```python
from build123d import *

# Parameters (mm, degrees)
F0_R      = 10
F1_DEPTH  = 5
F2_W      = 15.5
F2_H      = 10
F2_W_2    = 4
F3_DEPTH  = 5
F4_R      = 2.3
F5_DEPTH  = 22.751
F7_DEPTH  = 4
F8_R      = 2.3
F9_DEPTH  = 3
F10_R     = 2.3
F11_DEPTH = 3
F12_R     = 4.99999
F13_R     = 1
F14_DEPTH = 25
F15_R     = 1
F16_DEPTH = 25


# Not quite as in the source:
# - a fillet or chamfer is up to 0.001 mm smaller than in the source, because OpenCascade refuses the exact size


with BuildPart() as f1:
    # F0 (on Top) → F1 (new body)
    with BuildSketch(Plane.XY):
        with BuildLine():
            ThreePointArc((7.75, 12.842799539), (0, 15), (-7.75, 12.842799539))
            ThreePointArc((-7.75, 12.842799539), (-14.634921734, 3.289234841), (-12.5, -8.2915619759))
            ThreePointArc((-12.5, -8.2915619759), (-10.6951593818, -10.5172984077), (-8.5, -12.3592070943))
            ThreePointArc((-8.5, -12.3592070943), (0, -15), (8.5, -12.3592070943))
            ThreePointArc((8.5, -12.3592070943), (10.6951593818, -10.5172984077), (12.5, -8.2915619759))
            ThreePointArc((12.5, -8.2915619759), (14.3614066163, -4.3301270189), (15, 0))
            ThreePointArc((15, 0), (13.0623504776, 7.3739406019), (7.75, 12.842799539))
        make_face()
        Circle(F0_R, mode=Mode.SUBTRACT)
        with BuildLine():
            Line((-7.75, 26), (-7.75, 12.842799539))
            ThreePointArc((-7.75, 12.842799539), (0, 15), (7.75, 12.842799539))
            Line((7.75, 12.842799539), (7.75, 26))
            Line((7.75, 26), (-7.75, 26))
        make_face()
        with BuildLine():
            ThreePointArc((-8.5, -12.3592070943), (-10.6951593818, -10.5172984077), (-12.5, -8.2915619759))
            Line((-12.5, -8.2915619759), (-12.5, -26))
            Line((-12.5, -26), (-8.5, -26))
            Line((-8.5, -26), (-8.5, -12.3592070943))
        make_face()
        with BuildLine():
            ThreePointArc((12.5, -8.2915619759), (10.6951593818, -10.5172984077), (8.5, -12.3592070943))
            Line((8.5, -12.3592070943), (8.5, -26))
            Line((8.5, -26), (12.5, -26))
            Line((12.5, -26), (12.5, -8.2915619759))
        make_face()
    extrude(amount=F1_DEPTH)

    # F2 (on face) → F3 (join)
    with BuildSketch(Plane(origin=(0, 0, 0), x_dir=(1, 0, 0), z_dir=(0, 0, -1))):
        with Locations((0, -21)):
            Rectangle(F2_W, F2_H)
        with Locations((-10.5, 21)):
            Rectangle(F2_W_2, F2_H)
        with Locations((10.5, 21)):
            Rectangle(F2_W_2, F2_H)
    extrude(amount=F3_DEPTH)

    # F4 (on face) → F5 (cut, through all)
    with BuildSketch(Plane(origin=(-7.75, 0, 0), x_dir=(0, -1, 0), z_dir=(-1, 0, 0))):
        with Locations((-21, 0)):
            Circle(F4_R)
    extrude(amount=-F5_DEPTH, mode=Mode.SUBTRACT)

    # F6 (on face) → F7 (cut)
    with BuildSketch(Plane.XY.offset(5)):
        with BuildLine():
            ThreePointArc((10.4388347648, -8.8388347648), (9.4511282566, -7.3606275128), (7.7074639149, -7.7074639149))
            Line((7.7074639149, -7.7074639149), (9.9702056147, -9.9702056147))
            ThreePointArc((9.9702056147, -9.9702056147), (10.3170420168, -9.4511282566), (10.4388347648, -8.8388347648))
        make_face()
        with BuildLine():
            Line((9.9702056147, -9.9702056147), (7.7074639149, -7.7074639149))
            ThreePointArc((7.7074639149, -7.7074639149), (7.7074639149, -9.9702056147), (9.9702056147, -9.9702056147))
        make_face()
        with BuildLine():
            ThreePointArc((9.9702056147, 9.9702056147), (7.7074639149, 9.9702056147), (7.7074639149, 7.7074639149))
            Line((7.7074639149, 7.7074639149), (9.9702056147, 9.9702056147))
        make_face()
        with BuildLine():
            Line((9.9702056147, 9.9702056147), (7.7074639149, 7.7074639149))
            ThreePointArc((7.7074639149, 7.7074639149), (9.4511282566, 7.3606275128), (10.4388347648, 8.8388347648))
            ThreePointArc((10.4388347648, 8.8388347648), (10.3170420168, 9.4511282566), (9.9702056147, 9.9702056147))
        make_face()
        with BuildLine():
            ThreePointArc((-9.9702056147, 9.9702056147), (-9.9702056147, 7.7074639149), (-7.7074639149, 7.7074639149))
            Line((-7.7074639149, 7.7074639149), (-9.9702056147, 9.9702056147))
        make_face()
        with BuildLine():
            Line((-9.9702056147, 9.9702056147), (-7.7074639149, 7.7074639149))
            ThreePointArc((-7.7074639149, 7.7074639149), (-7.3606275128, 8.226541273), (-7.2388347648, 8.8388347648))
            ThreePointArc((-7.2388347648, 8.8388347648), (-8.226541273, 10.3170420168), (-9.9702056147, 9.9702056147))
        make_face()
        with BuildLine():
            ThreePointArc((-7.2388347648, -8.8388347648), (-7.3606275128, -8.226541273), (-7.7074639149, -7.7074639149))
            Line((-7.7074639149, -7.7074639149), (-9.9702056147, -9.9702056147))
            ThreePointArc((-9.9702056147, -9.9702056147), (-8.226541273, -10.3170420168), (-7.2388347648, -8.8388347648))
        make_face()
        with BuildLine():
            Line((-9.9702056147, -9.9702056147), (-7.7074639149, -7.7074639149))
            ThreePointArc((-7.7074639149, -7.7074639149), (-9.9702056147, -7.7074639149), (-9.9702056147, -9.9702056147))
        make_face()
    extrude(amount=-F7_DEPTH, mode=Mode.SUBTRACT)

    # F8 (on face) → F9 (cut)
    with BuildSketch(Plane.YZ.offset(-8.5)):
        with Locations((-21, 0)):
            Circle(F8_R)
    extrude(amount=-F9_DEPTH, mode=Mode.SUBTRACT)

    # F10 (on face) → F11 (cut)
    with BuildSketch(Plane(origin=(8.5, 0, 0), x_dir=(0, -1, 0), z_dir=(-1, 0, 0))):
        with Locations((21, 0)):
            Circle(F10_R)
    extrude(amount=-F11_DEPTH, mode=Mode.SUBTRACT)

    # F12 (radius 5 in the source; OpenCascade refuses exactly that, so slightly less here)
    f12_edges = [f1.edges().sort_by_distance(p)[0] for p in [
        (0, 26, -5),
        (0, 16, -5),
        (0, 26, 5),
        (-10.5, -26, -5),
        (-10.5, -26, 5),
        (10.5, -26, 5),
        (10.5, -26, -5),
        (-10.5, -16, -5),
        (10.5, -16, -5),
    ]]
    fillet(f12_edges, radius=F12_R)

    # F13 (on Right) → F14 (cut, symmetric)
    with BuildSketch(Plane.YZ):
        with Locations((0, 2.5)):
            Circle(F13_R)
    extrude(amount=F14_DEPTH, both=True, mode=Mode.SUBTRACT)

    # F15 (on Front) → F16 (cut)
    with BuildSketch(Plane.XZ):
        with Locations((0, 2.5)):
            Circle(F15_R)
    extrude(amount=F16_DEPTH, mode=Mode.SUBTRACT)


solid = f1.part
```
Can you work these out from the model? Positions are in its coordinate system, mm. A direction names the side the tool comes from. Coordinates: 2 decimals unless noted, no trailing zeros. Write each loop counter-clockwise with the first axis right and the second up, starting at its lowest first coordinate (ties: lowest second). Pieces come first, ordered by that corner, then holes. Notation, with made-up numbers: M -10,6 L 5,6 A14 ccw 5,16 Z; hole C -29.5,-6.75 d1. An arc over 180 degrees is marked long. Write item = value, one per line. Start each with the question number.
Q1. If we section it at A-A, the plane x = 0: State how many separate pieces and enclosed holes the cut face has, then the cut area to 3 significant figures.
Q2. I'm going to push flat-ended pins straight in: pin 1 (2 mm diameter, centred on x = -11, z = 0.5, fed in from +Y); pin 2 (5.5 mm diameter, centred on y = 21, z = 0, fed in from +X); pin 3 (1 mm diameter, centred on x = -8.5, y = 9, fed in from +Z); pin 4 (18 mm diameter, centred on x = 0, y = 0, fed in from +Z). Where does each tip first touch, or does it pass through?
Q3. If I drill on L1, parallel to Z at x = 0, y = -11.2; L2, parallel to X at y = 0.5, z = 4; L3, parallel to X at y = -17, z = -1, over which ranges is the centre line in solid material (lowest first)? Write a range as [from, to].
Q4. If we section it at C-C, the plane y = 5.5: Write out the boundary of the cut face in (x, z).
Q5. Thinking about a two-plate mould opening in X: for faces 5 (the face through (11.5, -21, 0)), 6 (the face through (-10, -25, -3)), 7 (the face through (-14.597, 3.454, 2.465)), which applies, released by +X, released by -X, zero draft, split by the parting line, or undercut?
Q6. If we section it at D-D, the plane z = 3: Write out the boundary of the cut face in (x, y), then the cut area to 3 significant figures.
Q7. On a 3-axis mill with a long thin cutter (end or side, diameter ignored), from which of +Z, -Z, +X, -X, +Y, -Y can I reach the whole of each face in a straight line? I mean faces 1 (the face through (7.75, 18, 1)), 2 (the face through (-12.5, -19, 1)), 3 (the face through (-0.13, -12.44, 3.49)), 4 (the face through (-9, 9, 1)). Say none if no direction works.
Check sheet entries:
q1.separate_pieces = 3
q1.enclosed_holes = 1
q1.area = 112 mm²
q2.pin_1 = 11.18
q2.pin_2 = 7.75
q2.pin_3 = 1
q2.pin_4 = through
q3.L1 = [0, 1.5], [3.5, 5]
q3.L2 = [-14.99, -9.99], [9.99, 14.99]
q3.L3 = [-12.5, -8.5], [8.5, 12.5]
q4.outline = M -13.96,0 L -8.35,0 L -8.35,5 L -13.96,5 Z; M 8.35,0 L 13.96,0 L 13.96,5 L 8.35,5 Z
q5.face_5 = undercut
q5.face_6 = zero draft
q5.face_7 = released by -X
q6.outline = M -14.97,-0.87 A15 ccw -12.5,-8.29 L -12.5,-25 L -8.5,-25 L -8.5,-12.36 A15 ccw -0.87,-14.97 L -0.87,-9.96 A10 cw -9.96,-0.87 Z; M -14.97,0.87 L -9.96,0.87 A10 cw 9.96,0.87 L 14.97,0.87 A15 ccw 7.75,12.84 L 7.75,25 L -7.75,25 L -7.75,12.84 A15 ccw Z; M 0.87,-14.97 A15 ccw 8.5,-12.36 L 8.5,-25 L 12.5,-25 L 12.5,-8.29 A15 ccw 14.97,-0.87 L 9.96,-0.87 A10 cw 0.87,-9.96 Z; hole C -8.84,-8.84 d3.2; hole C -8.84,8.84 d3.2; hole C 8.84,-8.84 d3.2; hole C 8.84,8.84 d3.2
q6.area = 616 mm²
q7.face_1 = +Z, -Z, +X, +Y
q7.face_2 = +Z, -Z, -X, -Y
q7.face_3 = -Y
q7.face_4 = +Z
